from build123d import *

# Parameters (mm, degrees)
SKETCH1_W           = 13
SKETCH1_H           = 18
BOSS_EXTRUDE1_DEPTH = 3.4
SKETCH2_W           = 15
SKETCH2_H           = 20
BOSS_EXTRUDE2_DEPTH = 1
SKETCH3_R           = 1.5
CUT_EXTRUDE1_DEPTH  = 14.251792332
FILLET1_R           = 0.2
FILLET2_R           = 1


with BuildPart() as part:
    # Sketch1 → Boss-Extrude1 (new body)
    with BuildSketch(Plane(origin=(0, 0, 0), x_dir=(1, 0, 0), z_dir=(0, 1, 0))):
        Rectangle(SKETCH1_W, SKETCH1_H)
    extrude(amount=BOSS_EXTRUDE1_DEPTH)

    # Sketch2 → Boss-Extrude2 (add)
    with BuildSketch(Plane(origin=(0, 3.4, 0), x_dir=(1, 0, 0), z_dir=(0, 1, 0))):
        Rectangle(SKETCH2_W, SKETCH2_H)
    extrude(amount=BOSS_EXTRUDE2_DEPTH)

    # Sketch3 → Cut-Extrude1 (cut, through all)
    with BuildSketch(Plane.XZ):
        with Locations(Location((0, 3, 0), (0, 0, 270))):
            Circle(SKETCH3_R)
        with Locations(Location((0, -3, 0), (0, 0, 270))):
            Circle(SKETCH3_R)
        Polygon((4.8, -5.5), (-1.3, -5.5), (-1.3, -5.9), (5.5, -5.9), (5.5, 8), (4.8, 8), align=None)
        Polygon((2.5, 7.85), (2.5, -4.3), (3.6, -4.3), (3.6, 8), (-5.5, 8), (-5.5, 7.6), (1.5, 7.6), (1.5, 7.85), align=None)
        Polygon((-2.5, -7.1), (-2.5, 4.3), (-3.9, 4.3), (-3.9, -8), (5.5, -8), (5.5, -7.1), align=None)
        Polygon((-5.35, 5.5), (1.3, 5.5), (1.3, 6.4), (-5.5, 6.4), (-5.5, -8), (-5.1, -8), (-5.1, 4.3), (-5.35, 4.3), align=None)
    extrude(amount=-CUT_EXTRUDE1_DEPTH, mode=Mode.SUBTRACT)

    # Fillet1
    fillet1_edges = [part.edges().sort_by_distance(p)[0] for p in [
        (-5.1, 2.2, -8),
        (-3.9, 2.2, -8),
        (-5.5, 2.2, 6.4),
        (-5.5, 2.2, 7.6),
        (4.8, 2.2, 8),
        (3.6, 2.2, 8),
        (-3.9, 2.2, 4.3),
        (-2.5, 2.2, 4.3),
        (1.3, 2.2, 5.5),
        (1.3, 2.2, 6.4),
        (5.5, 2.2, -7.1),
        (5.5, 2.2, -5.9),
        (-1.3, 2.2, -5.9),
        (-1.3, 2.2, -5.5),
        (3.6, 2.2, -4.3),
        (2.5, 2.2, -4.3),
    ]]
    fillet(fillet1_edges, radius=FILLET1_R - 0.0001)  # a hair under: the kernel refuses the full size

    # Fillet2
    fillet2_edges = [part.edges().sort_by_distance(p)[0] for p in [
        (6.5, 1.7, 9),
        (-6.5, 1.7, 9),
        (-6.5, 1.7, -9),
        (6.5, 1.7, -9),
    ]]
    fillet(fillet2_edges, radius=FILLET2_R)


solid = part.part
Geometry: final body of the model. Coordinates: model frame, mm. A direction names the side the tool comes from. Give positions to 0.01 mm unless a question says otherwise; leave off trailing zeros. Write each loop counter-clockwise with the first axis right and the second up, starting at its lowest first coordinate (ties: lowest second). Pieces come first, ordered by that corner, then holes.
(1) Cut plane A-A, the plane z = 7. Return loops of the section in (x, y).
(2) Access query for faces 5 (the flat face through (2.5, 2, 2)), 6 (the cylindrical face through (6.199, 1.724, -8.715)), 7 (the cylindrical face through (-6.215, 1.724, 8.699)), 8 (the flat face through (0, 2, 9)). Directions: +Z, -Z, +X, -X, +Y, -Y. A direction counts if a zero-diameter tool reaches every point of the face in a straight line with its end or side. Return the directions, or none.
(3) Mould query, pull axis Z, two halves, no side actions, for faces 1 (the flat face through (-5.1, 2, -2)), 2 (the flat face through (1, 2, -8)), 3 (the flat face through (0, 2, -9)), 4 (the flat face through (-7, 3.4, 0)). Classes: released by +Z, released by -Z, zero draft, split by the parting line, or undercut.
(4) Ray query, line 1 (X direction, y = 3.35, z = -0.25); line 2 (X direction, y = 1.1, z = -3); line 3 (X direction, y = 1.4, z = -7). Return the intervals inside material, ascending.
(5) First-contact query: P1, Ø1.7, axis at y = 2.5, z = 0.5, coming from the +X side; P2, Ø4, axis at x = 0, z = 3, coming from the -Y side; P3, Ø0.5, axis at x = -3, y = 2, coming from the -Z side; P4, Ø1.5, axis at y = 1.5, z = 7, coming from the -X side. Flat tips, straight axial feed; report the tip coordinate or a pass-through.
(6) Cut plane B-B, the plane z = -3. Return loops of the section in (x, y), then the cut area to 3 significant figures.
(7) Cut plane C-C, the plane x = 0. Give the number of separate pieces and of enclosed holes in the cut face, then the cut area to 3 significant figures.
Values follow:
1. outline: (-7.5, 3.4) - (-6.5, 3.4) - (-6.5, 0) - (2.5, 0) - (2.5, 4.4) - (-7.5, 4.4) - close; (3.6, 0) - (4.8, 0) - (4.8, 4.4) - (3.6, 4.4) - close; (5.5, 0) - (6.5, 0) - (6.5, 3.4) - (7.5, 3.4) - (7.5, 4.4) - (5.5, 4.4) - close
2. face 5: +Y, -Y
2. face 6: -Z, +X, -Y
2. face 7: +Z, -X, -Y
2. face 8: +Z, +X, -X, -Y
3. face 1: undercut
3. face 2: undercut
3. face 3: released by -Z
3. face 4: zero draft
4. line 1: x = -6.5 to -5.5, -5.1 to -3.9, -2.5 to 2.5, 3.6 to 4.8, 5.5 to 6.5
4. line 2: x = -6.5 to -5.5, -5.1 to -3.9, -2.5 to -1.5, 1.5 to 2.5, 3.6 to 4.8, 5.5 to 6.5
4. line 3: x = -6.5 to -5.5, -5.1 to -3.9, -2.5 to 6.5
5. P1: stops at x = 6.5
5. P2: stops at y = 0
5. P3: stops at z = -9
5. P4: stops at x = -6.5
6. outline: (-7.5, 3.4) - (-6.5, 3.4) - (-6.5, 0) - (-5.5, 0) - (-5.5, 4.4) - (-7.5, 4.4) - close; (-5.1, 0) - (-3.9, 0) - (-3.9, 4.4) - (-5.1, 4.4) - close; (-2.5, 0) - (-1.5, 0) - (-1.5, 4.4) - (-2.5, 4.4) - close; (1.5, 0) - (2.5, 0) - (2.5, 4.4) - (1.5, 4.4) - close; (3.6, 0) - (4.8, 0) - (4.8, 4.4) - (3.6, 4.4) - close; (5.5, 0) - (6.5, 0) - (6.5, 3.4) - (7.5, 3.4) - (7.5, 4.4) - (5.5, 4.4) - close
6. area: 30.2 mm2
7. separate pieces: 7
7. enclosed holes: 0
7. area: 43.4 mm2
